```python
from build123d import *

# Parameters (mm, degrees)
SKETCH_1_W          = 71
SKETCH_1_H          = 61.8
EXTRUDE_1_DEPTH     = 3
FILLET_1_R          = 5
FILLET_3_R          = 5
FILLET_4_R          = 5
SKETCH_2_R          = 1.5
CUT_EXTRUDE_1_DEPTH = 4
CUT_EXTRUDE_2_DEPTH = 4
SKETCH_6_W          = 27.5
SKETCH_6_H          = 27.5
CUT_EXTRUDE_3_DEPTH = 4
FILLET_5_R          = 5
FILLET_6_R          = 3
CUT_EXTRUDE_4_DEPTH = 4


with BuildPart() as part:
    # 草图1 → 凸台-拉伸1 (new body)
    with BuildSketch(Plane(origin=(0, 0, 0), x_dir=(1, 0, 0), z_dir=(0, 1, 0))):
        with Locations((-1.407488987, -9.162114537)):
            Rectangle(SKETCH_1_W, SKETCH_1_H)
    extrude(amount=EXTRUDE_1_DEPTH)

    # 圆角1
    fillet_1_edges = [part.edges().sort_by_distance(p)[0] for p in [
        (-36.907488987, 1.5, -21.737885463),
    ]]
    fillet(fillet_1_edges, radius=FILLET_1_R)

    # 圆角3
    fillet_3_edges = [part.edges().sort_by_distance(p)[0] for p in [
        (34.092511013, 1.5, 40.062114537),
    ]]
    fillet(fillet_3_edges, radius=FILLET_3_R)

    # 圆角4
    fillet_4_edges = [part.edges().sort_by_distance(p)[0] for p in [
        (34.092511013, 1.5, -21.737885463),
    ]]
    fillet(fillet_4_edges, radius=FILLET_4_R)

    # 草图2 → 切除-拉伸1 (cut, through all)
    with BuildSketch(Plane(origin=(0, 0, 0), x_dir=(-1, 0, 0), z_dir=(0, -1, 0))):
        with Locations((30.407488987, 15.237885463)):
            Circle(SKETCH_2_R)
        with Locations((-27.592511013, -33.562114537)):
            Circle(SKETCH_2_R)
        with Locations((-27.592511013, 15.237885463)):
            Circle(SKETCH_2_R)
    extrude(amount=-CUT_EXTRUDE_1_DEPTH, mode=Mode.SUBTRACT)

    # 草图5 → 切除-拉伸2 (cut, through all)
    with BuildSketch(Plane(origin=(0, 0, 0), x_dir=(-1, 0, 0), z_dir=(0, -1, 0))):
        with BuildLine():
            Line((24.407488987, 11.737885463), (-21.592511013, 11.737885463))
            ThreePointArc((-21.592511013, 11.737885463), (-25.092511013, 15.237885463), (-21.592511013, 18.737885463))
            Line((-21.592511013, 18.737885463), (24.407488987, 18.737885463))
            ThreePointArc((24.407488987, 18.737885463), (27.907488987, 15.237885463), (24.407488987, 11.737885463))
        make_face()
    extrude(amount=-CUT_EXTRUDE_2_DEPTH, mode=Mode.SUBTRACT)

    # 草图6 → 切除-拉伸3 (cut, through all)
    with BuildSketch(Plane.XZ):
        with Locations((-23.157488987, 26.312114537)):
            Rectangle(SKETCH_6_W, SKETCH_6_H)
    extrude(amount=-CUT_EXTRUDE_3_DEPTH, mode=Mode.SUBTRACT)

    # 圆角5
    fillet_5_edges = [part.edges().sort_by_distance(p)[0] for p in [
        (-36.907488987, 1.5, 12.562114537),
        (-9.407488987, 1.5, 40.062114537),
    ]]
    fillet(fillet_5_edges, radius=FILLET_5_R)

    # 圆角6
    fillet_6_edges = [part.edges().sort_by_distance(p)[0] for p in [
        (-9.407488987, 1.5, 12.562114537),
    ]]
    fillet(fillet_6_edges, radius=FILLET_6_R)

    # 草图7 → 切除-拉伸4 (cut, through all)
    with BuildSketch(Plane.XZ):
        with BuildLine():
            Line((3.592511013, 35.062114537), (18.592511013, 35.062114537))
            ThreePointArc((18.592511013, 35.062114537), (20.092511013, 33.562114537), (18.592511013, 32.062114537))
            Line((18.592511013, 32.062114537), (3.592511013, 32.062114537))
            ThreePointArc((3.592511013, 32.062114537), (2.092511013, 33.562114537), (3.592511013, 35.062114537))
        make_face()
    extrude(amount=-CUT_EXTRUDE_4_DEPTH, mode=Mode.SUBTRACT)


solid = part.part
```
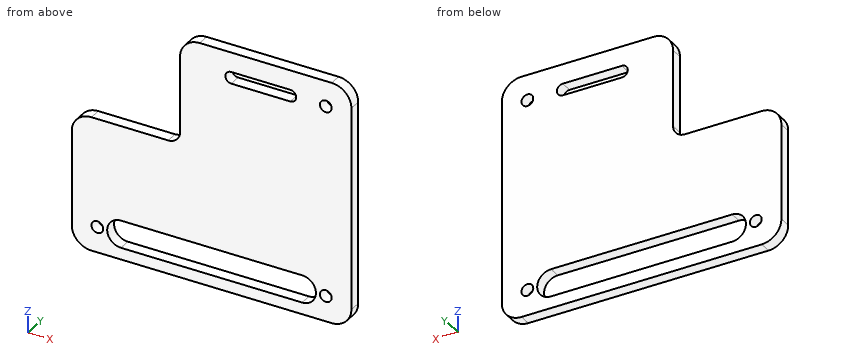
Verification items for the finished model (mm, model axes). Round coordinates to 2 decimals unless told otherwise and drop trailing zeros. Order: outer loops, then holes, each group sorted by start corner. A loop starts at its lowest first (then second) coordinate and runs counter-clockwise, first axis right, second up. Notation, with made-up numbers: (64.25, 52.5) -> (75.25, 52.5) arc R4 cw to (75.25, 57.5) -> close; hole circle Ø9 at (43.25, 49). An arc over 180 degrees is marked (long way). Put each result on its own line as item: value. Start each with the question number.
(1) Section check C-C (y = 2.15). Enter the section's corners in (x, z), then the cut area to 3 significant figures.
(2) Section check D-D (x = -8.5). Enter the section's corners in (y, z), then the cut area to 3 significant figures.
(3) Section check B-B (x = 14). Enter the section's corners in (y, z).
(4) Section check A-A (x = -23). Enter the section's corners in (y, z), then the cut area to 3 significant figures.
(5) Depth check by flat-ended pin: pin 1 Ø1.5 at (y, z) = (1.5, 23.5) entering from -X. Enter the tip coordinate at first touch or a pass-through.
(6) Material ranges on line 1 along Z through (x, y) = (3.5, 0.2); line 2 along Z through (x, y) = (27.5, 2.6); line 3 along Z through (x, y) = (-16.5, 1.45), recorded low to high.
Completed:
1. outline: (-36.91, -16.74) arc R5 ccw to (-31.91, -21.74) -> (29.09, -21.74) arc R5 ccw to (34.09, -16.74) -> (34.09, 35.06) arc R5 ccw to (29.09, 40.06) -> (-4.41, 40.06) arc R5 ccw to (-9.41, 35.06) -> (-9.41, 15.56) arc R3 cw to (-12.41, 12.56) -> (-31.91, 12.56) arc R5 ccw to (-36.91, 7.56) -> close; hole circle Ø3 at (-30.41, -15.24); hole (-24.41, -18.74) -> (21.59, -18.74) arc R3.5 ccw to (21.59, -11.74) -> (-24.41, -11.74) arc R3.5 ccw to start; hole (3.59, 32.06) -> (18.59, 32.06) arc R1.5 ccw to (18.59, 35.06) -> (3.59, 35.06) arc R1.5 ccw to start; hole circle Ø3 at (27.59, -15.24); hole circle Ø3 at (27.59, 33.56)
1. area: 3,170 mm2
2. outline: (0, -21.74) -> (3, -21.74) -> (3, -18.74) -> (0, -18.74) -> close; (0, -11.74) -> (3, -11.74) -> (3, 37.93) -> (0, 37.93) -> close
2. area: 158 mm2
3. outline: (0, -21.74) -> (3, -21.74) -> (3, -18.74) -> (0, -18.74) -> close; (0, -11.74) -> (3, -11.74) -> (3, 32.06) -> (0, 32.06) -> close; (0, 35.06) -> (3, 35.06) -> (3, 40.06) -> (0, 40.06) -> close
4. outline: (0, -21.74) -> (3, -21.74) -> (3, -18.74) -> (0, -18.74) -> close; (0, -11.74) -> (3, -11.74) -> (3, 12.56) -> (0, 12.56) -> close
4. area: 81.9 mm2
5. pin 1: stops at x = -9.41
6. line 1: z = -21.74 to -18.74, -11.74 to 32.06, 35.06 to 40.06
6. line 2: z = -21.74 to -16.74, -13.74 to 32.06, 35.06 to 40.06
6. line 3: z = -21.74 to -18.74, -11.74 to 12.56
